Source: CAD feature listing. Evaluate the final solid. Frame: model axes, mm. Face numbers are marked on the shaded views. A direction names the side the tool comes from. Give positions to 0.01 mm unless a question says otherwise; leave off trailing zeros. Write each loop counter-clockwise with the first axis right and the second up, starting at its lowest first coordinate (ties: lowest second). Pieces come first, ordered by that corner, then holes. Notation, with made-up numbers: (17.5, 7) -> (55.5, 7) arc R34 cw to (55.5, 38) -> close; hole circle Ø5 at (70.5, 83.5). An arc over 180 degrees is marked (long way). Answer as a JSON object with one key per item and string values. Group by question number.
Item 1: First-contact query: pin 1 Ø5 at (y, z) = (11, 4) entering from -X; pin 2 Ø4 at (y, z) = (14, 5) entering from +X (3 decimals); pin 3 Ø5 at (x, z) = (22, 7.5) entering from +Y (3 decimals). Flat tips, straight axial feed; report the tip coordinate or a pass-through.
Item 2: Section query C-C on y = 6.25. Return the cut outline in (x, z) (3 decimals).
Item 3: Section query B-B on x = 17. Return the cut outline in (y, z) (3 decimals).
Item 4: Pull-direction query (Y, two-part tool) for the marked faces 3, 4 and 5; classes: pulls with the +Y half, pulls with the -Y half, needs draft (parallel to the pull), parting line crosses it, or undercut.
Item 5: Access query for the marked faces 1 and 2. Directions: +Z, -Z, +X, -X, +Y, -Y. A direction counts if a zero-diameter tool reaches every point of the face in a straight line with its end or side. Return the directions, or none.
Item 6: Ray query, probe 1 along X at (y, z) = (2.55, 6.35); probe 2 along Y at (x, z) = (11.5, 4.5) (3 decimals). Return the intervals inside material, ascending. Write a range as from..to.
Item 7: Section query A-A on z = 6.35. Return the cut outline in (x, y) (3 decimals), plus the area to 3 significant figures.
from build123d import *

# Parameters (mm, degrees)
BOSS_EXTRUDE1_DEPTH = 12.7
SKETCH2_R           = 3.175
CUT_EXTRUDE1_DEPTH  = 4.175
SKETCH3_R           = 3.175
CUT_EXTRUDE2_DEPTH  = 4.175


with BuildPart() as part:
    # Sketch1 → Boss-Extrude1 (new body)
    with BuildSketch(Plane.XY):
        Polygon((0, 0), (0, 25.4), (3.175, 25.4), (3.175, 3.175), (38.1, 3.175), (38.1, 0), align=None)
    extrude(amount=BOSS_EXTRUDE1_DEPTH)

    # Sketch2 → Cut-Extrude1 (cut, through all)
    with BuildSketch(Plane(origin=(0, 3.175, 0), x_dir=(1, 0, 0), z_dir=(0, 1, 0))):
        with Locations((15.875, -6.35)):
            Circle(SKETCH2_R)
        with Locations((28.575, -6.35)):
            Circle(SKETCH2_R)
    extrude(amount=-CUT_EXTRUDE1_DEPTH, mode=Mode.SUBTRACT)

    # Sketch3 → Cut-Extrude2 (cut, through all)
    with BuildSketch(Plane(origin=(3.175, 0, 0), x_dir=(0, 0, -1), z_dir=(1, 0, 0))):
        with Locations((-6.35, 28.575)):
            Circle(SKETCH3_R)
        with Locations((-6.35, 15.875)):
            Circle(SKETCH3_R)
    extrude(amount=-CUT_EXTRUDE2_DEPTH, mode=Mode.SUBTRACT)


solid = part.part
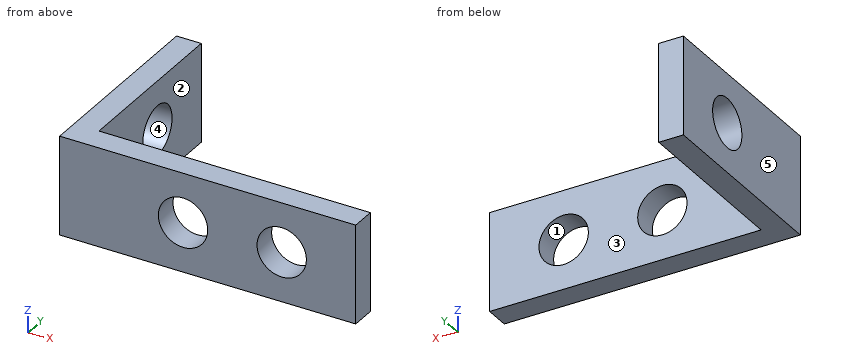
Worked answers:
{
 "1": {"pin 1": "x = 0", "pin 2": "x = 3.175", "pin 3": "y = 3.175"},
 "2": {"outline": "(0, 0) -> (3.175, 0) -> (3.175, 12.7) -> (0, 12.7) -> close"},
 "3": {"outline": "(0, 0) -> (3.175, 0) -> (3.175, 3.381) -> (0, 3.381) -> close; (0, 9.319) -> (3.175, 9.319) -> (3.175, 12.7) -> (0, 12.7) -> close"},
 "4": {"face 3": "pulls with the +Y half", "face 4": "undercut", "face 5": "needs draft"},
 "5": {"face 1": "+Y, -Y", "face 2": "+Z, -Z, +X, +Y"},
 "6": {"probe 1": "0..12.7, 19.05..25.4, 31.75..38.1", "probe 2": "0..3.175"},
 "7": {"outline": "(0, 0) -> (12.7, 0) -> (12.7, 3.175) -> (3.175, 3.175) -> (3.175, 12.7) -> (0, 12.7) -> close; (0, 19.05) -> (3.175, 19.05) -> (3.175, 25.4) -> (0, 25.4) -> close; (19.05, 0) -> (25.4, 0) -> (25.4, 3.175) -> (19.05, 3.175) -> close; (31.75, 0) -> (38.1, 0) -> (38.1, 3.175) -> (31.75, 3.175) -> close", "area": "131 mm^2"}
}
